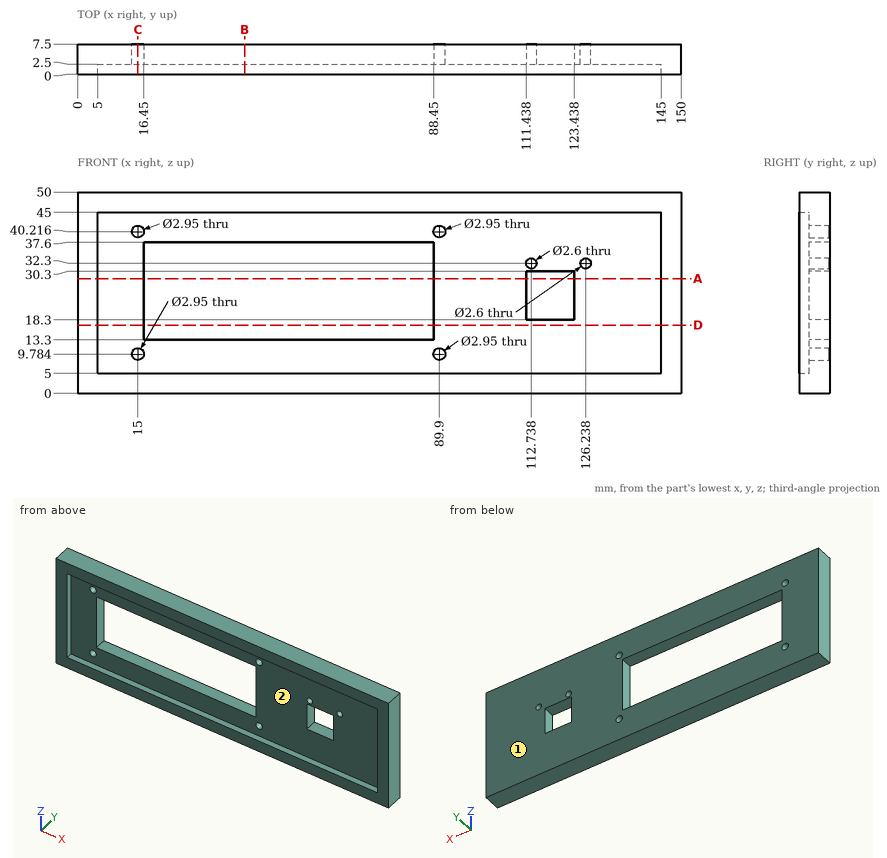
Job drawing, mm, ordinate dimensions from the low corner. One solid piece. Coordinates: 2 decimals unless noted, no trailing zeros. Loops run counter-clockwise (first coordinate to the right, second up) from the corner with the lowest first, then second, coordinate; pieces in that order, holes last. Notation, with made-up numbers: (-5, 70.5) - (45, 70.5) arc R10 cw to (45, 77.5) - close; hole circle Ø8 at (-19.75, 4.5). An arc over 180 degrees is marked (long way). Answer as a JSON object with one key per item and string values. Group by question number.
(1) Cut at D-D (z = 17). Give the cut face in (x, y), then the cut area to 3 significant figures.
(2) Probe line 1 along Z through (x, y) = (89.9, 4.05); line 2 along X through (y, z) = (5.25, 20); line 3 along X through (y, z) = (4.8, 32.3). List the from-to ranges inside material, lowest first.
(3) Cut at C-C (x = 15). Give the cut face in (y, z).
(4) Flat gauge pin, fed straight in: pin 1 (20 mm diameter, centred on x = 72.5, z = 18, fed in from -Y). Where does the tip first touch, or does it go through?
(5) Cut at B-B (x = 41.5). Give the cut face in (y, z).
(6) Two-plate mould, pull along X, no slides. Class the marked faces 1 and 2: released by +X, released by -X, zero draft, split by the parting line, or undercut.
(7) Cut at A-A (z = 28.5). Give the cut face in (x, y).
Geometry says:
{
 "1": {"outline": "(0, 0) - (5, 0) - (5, 2.5) - (16.45, 2.5) - (16.45, 7.5) - (0, 7.5) - close; (88.45, 2.5) - (145, 2.5) - (145, 0) - (150, 0) - (150, 7.5) - (88.45, 7.5) - close", "area": "415 mm^2"},
 "2": {"line 1": "z = 0 to 8.31, 11.26 to 38.74, 41.69 to 50", "line 2": "x = 0 to 16.45, 88.45 to 111.44, 123.44 to 150", "line 3": "x = 0 to 16.45, 88.45 to 111.44, 114.04 to 124.94, 127.54 to 150"},
 "3": {"outline": "(0, 0) - (7.5, 0) - (7.5, 8.31) - (2.5, 8.31) - (2.5, 5) - (0, 5) - close; (0, 45) - (2.5, 45) - (2.5, 41.69) - (7.5, 41.69) - (7.5, 50) - (0, 50) - close; (2.5, 11.26) - (7.5, 11.26) - (7.5, 38.74) - (2.5, 38.74) - close"},
 "4": {"pin 1": "stops at y = 2.5"},
 "5": {"outline": "(0, 0) - (7.5, 0) - (7.5, 13.3) - (2.5, 13.3) - (2.5, 5) - (0, 5) - close; (0, 45) - (2.5, 45) - (2.5, 37.6) - (7.5, 37.6) - (7.5, 50) - (0, 50) - close"},
 "6": {"face 1": "zero draft", "face 2": "undercut"},
 "7": {"outline": "(0, 0) - (5, 0) - (5, 2.5) - (16.45, 2.5) - (16.45, 7.5) - (0, 7.5) - close; (88.45, 2.5) - (111.44, 2.5) - (111.44, 7.5) - (88.45, 7.5) - close; (123.44, 2.5) - (145, 2.5) - (145, 0) - (150, 0) - (150, 7.5) - (123.44, 7.5) - close"}
}
